Read the model definition and answer for the solid it produces. Units are mm, in the model's axes. Coordinates: 2 decimals unless noted, no trailing zeros. Loops run counter-clockwise (first coordinate to the right, second up) from the corner with the lowest first, then second, coordinate; pieces in that order, holes last. Notation, with made-up numbers: (59.25, 1.25) -> (91.25, 1.25) arc R29 cw to (91.25, 36.25) -> close; hole circle Ø6 at (-31, -32.5). An arc over 180 degrees is marked (long way). Answer as CSV lines item,"result".
```python
from build123d import *

# Parameters (mm, degrees)
SKETCH1_W           = 132
SKETCH1_H           = 132
SKETCH1_R           = 2.5
SKETCH1_R_2         = 11
BOSS_EXTRUDE1_DEPTH = 1
SKETCH2_R           = 2
CUT_EXTRUDE1_DEPTH  = 2


with BuildPart() as part:
    # Sketch1 → Boss-Extrude1 (new body)
    with BuildSketch(Plane(origin=(0, 0, 0), x_dir=(1, 0, 0), z_dir=(0, 1, 0))):
        with Locations((39.311456102, 43.795094937)):
            Rectangle(SKETCH1_W, SKETCH1_H)
        with Locations((14.311456102, 29.795094937)):
            Circle(SKETCH1_R, mode=Mode.SUBTRACT)
        with Locations((24.311456102, 29.795094937)):
            Circle(SKETCH1_R, mode=Mode.SUBTRACT)
        with Locations((54.311456102, 29.795094937)):
            Circle(SKETCH1_R, mode=Mode.SUBTRACT)
        with Locations((64.311456102, 29.795094937)):
            Circle(SKETCH1_R, mode=Mode.SUBTRACT)
        with Locations((19.311456102, 49.795094937)):
            Circle(SKETCH1_R_2, mode=Mode.SUBTRACT)
        with Locations((59.311456102, 49.795094937)):
            Circle(SKETCH1_R_2, mode=Mode.SUBTRACT)
    extrude(amount=BOSS_EXTRUDE1_DEPTH)

    # Sketch2 → Cut-Extrude1 (cut, through all)
    with BuildSketch(Plane.XZ):
        with Locations((-10.688543898, -3.795094937)):
            Circle(SKETCH2_R)
        with Locations((89.311456102, -3.795094937)):
            Circle(SKETCH2_R)
        with Locations((89.311456102, -83.795094937)):
            Circle(SKETCH2_R)
        with Locations((-10.688543898, -83.795094937)):
            Circle(SKETCH2_R)
    extrude(amount=-CUT_EXTRUDE1_DEPTH, mode=Mode.SUBTRACT)


solid = part.part
```
Q1. Find the intervals of material crossed by probe 1 along Z at (x, y) = (55, 0.6); probe 2 along X at (y, z) = (0.1, -51); probe 3 along Z at (x, y) = (59, 0.4), in increasing order. Write a range as [from, to].
Results:
probe 1,"z = [-109.8, -59.91], [-39.68, -32.2], [-27.39, 22.2]"
probe 2,"x = [-26.69, 8.38], [30.25, 48.38], [70.25, 105.31]"
probe 3,"z = [-109.8, -60.79], [-38.8, 22.2]"
Q2. A cutting plane is placed at A-A, the plane z = -56.5. Write down the section's boundary in (x, y), and give its area (3 significant figures).
Results:
outline,"(-26.69, 0) -> (10.59, 0) -> (10.59, 1) -> (-26.69, 1) -> close; (28.03, 0) -> (50.59, 0) -> (50.59, 1) -> (28.03, 1) -> close; (68.03, 0) -> (105.31, 0) -> (105.31, 1) -> (68.03, 1) -> close"
area,"97.1 mm²"
Q3. Given pin 1 Ø3 at (x, z) = (54.31, -29.8) entering from -Y, flat-ended and moving along its own axis, determine where the tip first touches the part or whether it passes through.
Results:
pin 1,"passes through"
Q4. A cutting plane is placed at B-B, the plane y = 0.25. Give the number of separate pieces and of enclosed holes in the cut face, and give its area (3 significant figures).
Results:
separate pieces,"1"
enclosed holes,"10"
area,"16,500 mm²"
Q5. For a pull along Z with two mould halves and no side action, classify faces 1 (the face through (38, 0, -45)), 2 (the face through (15.47, 0.49, -27.58)) as pulls with the +Z half, pulls with the -Z half, needs draft (parallel to the pull), parting line crosses it, or undercut.
Results:
face 1,"needs draft"
face 2,"undercut"
